For this review, take the finished solid that the model builds, in its own axes (mm). Give positions to 0.01 mm unless a question says otherwise; leave off trailing zeros. Write each loop counter-clockwise with the first axis right and the second up, starting at its lowest first coordinate (ties: lowest second). Pieces come first, ordered by that corner, then holes. Notation, with made-up numbers: (89, 87) -> (120, 87) arc R21 ccw to (120, 124) -> close; hole circle Ø10 at (59, 9.5). An arc over 180 degrees is marked (long way). Answer as CSV lines item,"result".
```python
from build123d import *

# Parameters (mm, degrees)
SKETCH1_W          = 3.5
SKETCH1_H          = 6.65
CUT_EXTRUDE1_DEPTH = 9
CUT_EXTRUDE3_DEPTH = 10


with BuildPart() as part:
    # Sketch1 → Revolve1 (revolve)
    with BuildSketch(Plane(origin=(0, 0, 0), x_dir=(1, 0, 0), z_dir=(0, 1, 0))):
        with Locations((1.75, -3.325)):
            Rectangle(SKETCH1_W, SKETCH1_H)
    revolve(axis=Axis((0, 0, 0), (0, 0, 1)))

    # Sketch3 → Cut-Extrude1 (cut)
    with BuildSketch(Plane.XY.offset(6.65)):
        Polygon((2.06028803, 1.324066719), (1.700436542, 1.473436651), (1.603799186, 1.850882928), (1.216441839, 1.892820449), (1.017380071, 2.227751609), (0.633898253, 2.158859191), (0.348538872, 2.424141105), (0, 2.25), (-0.348538872, 2.424141105), (-0.633898253, 2.158859191), (-1.017380071, 2.227751609), (-1.216441839, 1.892820449), (-1.603799186, 1.850882928), (-1.700436542, 1.473436651), (-2.06028803, 1.324066719), (-2.04667199, 0.934683779), (-2.34986459, 0.689982499), (-2.227098244, 0.320208386), (-2.449069097, 0), (-2.227098244, -0.320208386), (-2.34986459, -0.689982499), (-2.04667199, -0.934683779), (-2.06028803, -1.324066719), (-1.700436542, -1.473436651), (-1.603799186, -1.850882928), (-1.216441839, -1.892820449), (-1.017380071, -2.227751609), (-0.633898253, -2.158859191), (-0.348538872, -2.424141105), (0, -2.25), (0.348538872, -2.424141105), (0.633898253, -2.158859191), (1.017380071, -2.227751609), (1.216441839, -1.892820449), (1.603799186, -1.850882928), (1.700436542, -1.473436651), (2.06028803, -1.324066719), (2.04667199, -0.934683779), (2.34986459, -0.689982499), (2.227098244, -0.320208386), (2.449069097, 0), (2.227098244, 0.320208386), (2.34986459, 0.689982499), (2.04667199, 0.934683779), align=None)
    extrude(amount=-CUT_EXTRUDE1_DEPTH, mode=Mode.SUBTRACT)

    # Sketch9 → Cut-Extrude3 (cut)
    with BuildSketch(Plane.XY.offset(6.65)):
        Polygon((0, -2.25), (0.383171844, -2.665018714), (0.633898253, -2.158859191), (1.118473228, -2.449114747), (1.216441839, -1.892820449), (1.763162563, -2.034798069), (1.700436542, -1.473436651), (2.265010954, -1.455634153), (2.04667199, -0.934683779), (2.583361627, -0.758543414), (2.227098244, -0.320208386), (2.692423705, 0), (2.227098244, 0.320208386), (2.583361627, 0.758543414), (2.04667199, 0.934683779), (2.265010954, 1.455634153), (1.700436542, 1.473436651), (1.763162563, 2.034798069), (1.216441839, 1.892820449), (1.118473228, 2.449114747), (0.633898253, 2.158859191), (0.383171844, 2.665018714), (0, 2.25), (-0.383171844, 2.665018714), (-0.633898253, 2.158859191), (-1.118473228, 2.449114747), (-1.216441839, 1.892820449), (-1.763162563, 2.034798069), (-1.700436542, 1.473436651), (-2.265010954, 1.455634153), (-2.04667199, 0.934683779), (-2.583361627, 0.758543414), (-2.227098244, 0.320208386), (-2.692423705, 0), (-2.227098244, -0.320208386), (-2.583361627, -0.758543414), (-2.04667199, -0.934683779), (-2.265010954, -1.455634153), (-1.700436542, -1.473436651), (-1.763162563, -2.034798069), (-1.216441839, -1.892820449), (-1.118473228, -2.449114747), (-0.633898253, -2.158859191), (-0.383171844, -2.665018714), align=None)
    extrude(amount=-CUT_EXTRUDE3_DEPTH, mode=Mode.SUBTRACT)


solid = part.part
```
Q1. Clearance check with flat-ended pins moving along their axes: pin 1 (1 mm diameter, centred on x = -1, y = 1, fed in from -Z); pin 2 (3 mm diameter, centred on y = 2, z = 1, fed in from +X). State where each tip first meets the part, or that it passes through.
Answer block:
pin 1,"passes through"
pin 2,"stops at x = 3.46"
Q2. Add section A-A (x = -0.25). Write out the cut boundary in (y, z), plus the area to 3 significant figures.
Answer block:
outline,"(-3.49, 0) -> (-2.52, 0) -> (-2.52, 6.65) -> (-3.49, 6.65) -> close; (2.52, 0) -> (3.49, 0) -> (3.49, 6.65) -> (2.52, 6.65) -> close"
area,"12.9 mm2"
Q3. Add section B-B (y = -0.5). Write out the cut boundary in (x, z), plus the area to 3 significant figures.
Answer block:
outline,"(-3.46, 0) -> (-2.37, 0) -> (-2.37, 6.65) -> (-3.46, 6.65) -> close; (2.37, 0) -> (3.46, 0) -> (3.46, 6.65) -> (2.37, 6.65) -> close"
area,"14.5 mm2"
Q4. To check wall thickness, follow probe 1 along X at (y, z) = (0.25, 4.5); probe 2 along X at (y, z) = (1.25, 5); probe 3 along Y at (x, z) = (-1, 1.25). State the ranges of each line that lie inside material, in increasing order. Write a range as [from, to].
Answer block:
probe 1,"x = [-3.49, -2.33], [2.33, 3.49]"
probe 2,"x = [-3.27, -2.18], [2.18, 3.27]"
probe 3,"y = [-3.35, -2.38], [2.38, 3.35]"
Q5. Add section C-C (y = -3). Write out the cut boundary in (x, z), plus the area to 3 significant figures.
Answer block:
outline,"(-1.8, 0) -> (1.8, 0) -> (1.8, 6.65) -> (-1.8, 6.65) -> close"
area,"24.0 mm2"
